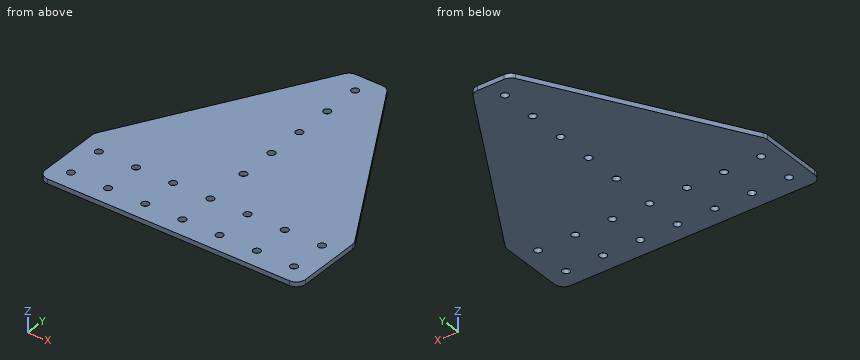
```python
from build123d import *

# Parameters (mm, degrees)
BOSS_EXTRUDE1_DEPTH = 3.175
SKETCH2_R           = 2.4892
CUT_EXTRUDE1_DEPTH  = 255.856797106
FILLET1_R           = 6.35


with BuildPart() as part:
    # Sketch1 → Boss-Extrude1 (new body)
    with BuildSketch(Plane.XY):
        Polygon((0, 0), (0, 50.8), (76.2, 182.5625), (101.6, 182.5625), (177.8, 50.8), (177.8, 0), align=None)
    extrude(amount=-BOSS_EXTRUDE1_DEPTH)

    # Sketch2 → Cut-Extrude1 (cut, through all)
    with BuildSketch(Plane.XY):
        with Locations((12.7, 12.7)):
            Circle(SKETCH2_R)
        with Locations((38.1, 12.7)):
            Circle(SKETCH2_R)
        with Locations((63.5, 12.7)):
            Circle(SKETCH2_R)
        with Locations((88.9, 12.7)):
            Circle(SKETCH2_R)
        with Locations((114.3, 12.7)):
            Circle(SKETCH2_R)
        with Locations((139.7, 12.7)):
            Circle(SKETCH2_R)
        with Locations((165.1, 12.7)):
            Circle(SKETCH2_R)
        with Locations((38.1, 38.1)):
            Circle(SKETCH2_R)
        with Locations((63.5, 38.1)):
            Circle(SKETCH2_R)
        with Locations((88.9, 38.1)):
            Circle(SKETCH2_R)
        with Locations((114.3, 38.1)):
            Circle(SKETCH2_R)
        with Locations((139.7, 38.1)):
            Circle(SKETCH2_R)
        with Locations((165.1, 38.1)):
            Circle(SKETCH2_R)
        with Locations((12.7, 38.1)):
            Circle(SKETCH2_R)
        with Locations((88.9, 169.8625)):
            Circle(SKETCH2_R)
        with Locations((88.9, 144.4625)):
            Circle(SKETCH2_R)
        with Locations((88.9, 119.0625)):
            Circle(SKETCH2_R)
        with Locations((88.9, 93.6625)):
            Circle(SKETCH2_R)
        with Locations((88.9, 68.2625)):
            Circle(SKETCH2_R)
    extrude(amount=-CUT_EXTRUDE1_DEPTH, mode=Mode.SUBTRACT)

    # Fillet1
    fillet1_edges = [part.edges().sort_by_distance(p)[0] for p in [
        (0, 0, -1.5875),
        (177.8, 0, -1.5875),
        (177.8, 50.8, -1.5875),
        (101.6, 182.5625, -1.5875),
        (76.2, 182.5625, -1.5875),
        (0, 50.8, -1.5875),
    ]]
    fillet(fillet1_edges, radius=FILLET1_R)


solid = part.part
```
The listing builds one solid part. Answer for the finished solid, in the listing's coordinates (mm). Give positions to 0.01 mm unless a question says otherwise; leave off trailing zeros. Order: outer loops, then holes, each group sorted by start corner. A loop starts at its lowest first (then second) coordinate and runs counter-clockwise, first axis right, second up. Notation, with made-up numbers: (-3, -31.5) -> (24, -31.5) arc R30 ccw to (24, -0.5) -> close; hole circle Ø9 at (49.5, 18). An arc over 180 degrees is marked (long way). Write each question's results on one line, items separated by ' | '.
Q1. Straight lines are drawn through the part: probe 1 along Y at (x, z) = (139.7, -2.15); probe 2 along Y at (x, z) = (12.7, -2.1); probe 3 along X at (y, z) = (66, -0.3). For each, find the intervals that lie inside material, in ascending order. Write a range as from..to.
Checked values:
probe 1: y = 0..10.21, 15.19..35.61, 40.59..116.68 | probe 2: y = 0..10.21, 15.19..35.61, 40.59..72.76 | probe 3: x = 8.79..87.86, 89.94..169.01
Q2. The part is cut by section A-A, the plane x = 88.9. State how many separate pieces and enclosed holes the cut face has, and give its area (3 significant figures).
Checked values:
separate pieces: 8 | enclosed holes: 0 | area: 469 mm^2
Q3. Each of these flat-tipped pins is pushed along its axis until it touches: P1, Ø1, axis at y = 161.5, z = -2.5, coming from the -X side; P2, Ø1.5, axis at y = 100.5, z = -0.5, coming from the +X side. Where does it stop, or does it pass through?
Checked values:
P1: stops at x = 63.73 | P2: stops at x = 149.49
Q4. The part is cut by section D-D, the plane x = 63.5. Give the vertices of the cut face in (y, z) (3 decimals), and give its area (3 significant figures).
Checked values:
outline: (0, -3.175) -> (10.211, -3.175) -> (10.211, 0) -> (0, 0) -> close; (15.189, -3.175) -> (35.611, -3.175) -> (35.611, 0) -> (15.189, 0) -> close; (40.589, -3.175) -> (160.602, -3.175) -> (160.602, 0) -> (40.589, 0) -> close | area: 478 mm^2
